```python
from build123d import *

# Parameters (mm, degrees)
SKETCH_1_W          = 140
SKETCH_1_H          = 125
EXTRUDE_1_DEPTH     = 2
SKETCH_3_R          = 2.2
CUT_EXTRUDE_1_DEPTH = 2
SKETCH_6_R          = 2.2
CUT_EXTRUDE_2_DEPTH = 2
SKETCH_7_R          = 2.2
CUT_EXTRUDE_3_DEPTH = 105


with BuildPart() as part:
    # ｽｹｯﾁ1 → ﾎﾞｽ - 押し出し1 (new body)
    with BuildSketch(Plane.XY):
        Rectangle(SKETCH_1_W, SKETCH_1_H)
    extrude(amount=EXTRUDE_1_DEPTH)

    # ｽｹｯﾁ3 → ｶｯﾄ - 押し出し1 (cut)
    with BuildSketch(Plane.XY.offset(2)):
        with Locations((-60, 54.5)):
            Circle(SKETCH_3_R)
        with Locations((-60, -51.5)):
            Circle(SKETCH_3_R)
    extrude(amount=-CUT_EXTRUDE_1_DEPTH, mode=Mode.SUBTRACT)

    # ｽｹｯﾁ6 → ｶｯﾄ - 押し出し2 (cut)
    with BuildSketch(Plane.XY.offset(2)):
        with Locations((62.5, -52.5)):
            Circle(SKETCH_6_R)
        with Locations((62.5, 47.5)):
            Circle(SKETCH_6_R)
    extrude(amount=-CUT_EXTRUDE_2_DEPTH, mode=Mode.SUBTRACT)

    # ｽｹｯﾁ7 → ｶｯﾄ - 押し出し3 (cut)
    with BuildSketch(Plane.XY.offset(2)):
        with BuildLine():
            ThreePointArc((42.8, 55), (45, 52.8), (47.2, 55))
            Line((47.2, 55), (45, 55))
            Line((45, 55), (42.8, 55))
        make_face()
        with BuildLine():
            Line((45, 55), (47.2, 55))
            ThreePointArc((47.2, 55), (45, 57.2), (42.8, 55))
            Line((42.8, 55), (45, 55))
        make_face()
        with Locations((-20, 55)):
            Circle(SKETCH_7_R)
        with Locations((-20, -55)):
            Circle(SKETCH_7_R)
        with Locations((45, -55)):
            Circle(SKETCH_7_R)
    extrude(amount=-CUT_EXTRUDE_3_DEPTH, mode=Mode.SUBTRACT)


solid = part.part
```
Part model, mm, in its own coordinate system. Round coordinates to 2 decimals unless told otherwise and drop trailing zeros. Write each loop counter-clockwise with the first axis right and the second up, starting at its lowest first coordinate (ties: lowest second). Pieces come first, ordered by that corner, then holes.
Item 1: Cut at B-B, the plane y = 47.5. Give the cut face in (x, z).
Results:
outline: (-70, 0) - (60.3, 0) - (60.3, 2) - (-70, 2) - close; (64.7, 0) - (70, 0) - (70, 2) - (64.7, 2) - close
Item 2: Two-plate mould, pull along X, no slides. Class faces 1 (the flat face through (-1, 1, 2)), 2 (the cylindrical face through (63.52, 45.55, 1.01)): +X half, -X half, draft (parallel to the pull), parting line (faces both ways), or undercut.
Results:
face 1: draft
face 2: undercut
Item 3: Drop a flat-ended pin along its axis: pin 1 Ø4 at (x, y) = (45, 55) entering from -Z. Give the stop position or say it passes through.
Results:
pin 1: passes through
Item 4: Probe L1, parallel to Y at x = 45, z = 1.4; L2, parallel to Y at x = -60, z = 0.75. List the from-to ranges inside material, lowest first.
Results:
L1: y = -62.5 to -57.2, -52.8 to 52.8, 57.2 to 62.5
L2: y = -62.5 to -53.7, -49.3 to 52.3, 56.7 to 62.5
Item 5: Cut at A-A, the plane x = 45. Give the cut face in (y, z).
Results:
outline: (-62.5, 0) - (-57.2, 0) - (-57.2, 2) - (-62.5, 2) - close; (-52.8, 0) - (52.8, 0) - (52.8, 2) - (-52.8, 2) - close; (57.2, 0) - (62.5, 0) - (62.5, 2) - (57.2, 2) - close
